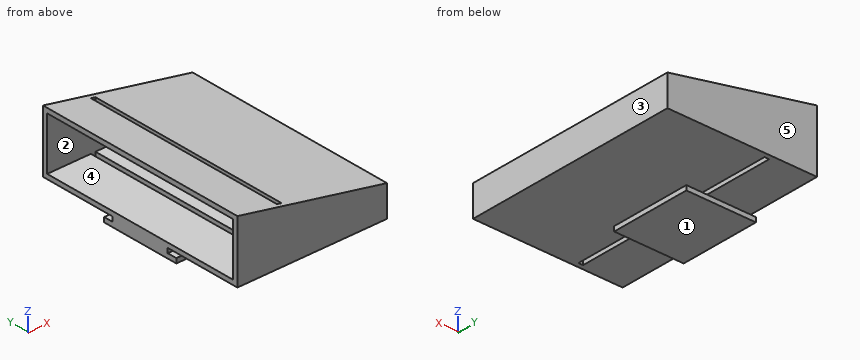
from build123d import *

# Parameters (mm, degrees)
SKETCH1_W           = 2.9
SKETCH1_H           = 19.8
BOSS_EXTRUDE1_DEPTH = 1.5
SKETCH2_W           = 22.5
SKETCH2_H           = 26
BOSS_EXTRUDE3_DEPTH = 1.5
BOSS_EXTRUDE4_DEPTH = 20
CUT_EXTRUDE1_DEPTH  = 70
CUT_EXTRUDE2_START  = -35
CUT_EXTRUDE2_DEPTH  = 33.5
CUT_EXTRUDE3_REACH  = 80.921
SKETCH6_W           = 1.5
SKETCH6_H           = 67


with BuildPart() as part:
    # Sketch1 → Boss-Extrude1 (new body)
    with BuildSketch(Plane.XY):
        with Locations((-45.437495374, 25.25)):
            Rectangle(SKETCH1_W, SKETCH1_H)
    extrude(amount=-BOSS_EXTRUDE1_DEPTH)

    # Sketch2 → Boss-Extrude3 (add)
    with BuildSketch(Plane(origin=(0, 0, -1.5), x_dir=(-1, 0, 0), z_dir=(0, 0, -1))):
        with Locations((35.637495374, 25.25)):
            Rectangle(SKETCH2_W, SKETCH2_H)
    extrude(amount=BOSS_EXTRUDE3_DEPTH)

    # Sketch3 → Boss-Extrude4 (add)
    with BuildSketch(Plane.XY):
        Polygon((-46.887495374, 15.25), (-46.887495374, 35.25), (-46.887495374, 60.25), (1.5, 60.25), (1.5, -9.75), (-46.887495374, -9.75), align=None)
    extrude(amount=BOSS_EXTRUDE4_DEPTH)

    # Sketch4 → Cut-Extrude1 (cut)
    with BuildSketch(Plane.XZ.offset(9.75)):
        Polygon((-46.887495374, 20), (1.5, 10), (1.5, 20), align=None)
    extrude(amount=-CUT_EXTRUDE1_DEPTH, mode=Mode.SUBTRACT)

    # Sketch5 → Cut-Extrude2 (cut)
    with BuildSketch(Plane.XZ.offset(9.75).offset(CUT_EXTRUDE2_START)):
        Polygon((0, 1.5), (0, 8.778299559), (-46.887495374, 18.468302113), (-46.887495374, 1.5), align=None)
    cut_extrude2 = extrude(amount=CUT_EXTRUDE2_DEPTH, mode=Mode.SUBTRACT)

    # Mirror1: Cut-Extrude2 across plane
    add(cut_extrude2.mirror(Plane.ZX.offset(25.25)), mode=Mode.SUBTRACT)

    # Cut-Extrude3: up to this plane
    cut_extrude3_end = Plane(origin=(-46.887495374, 109.660016278, 20), z_dir=(-0.20238811385578315, 0, -0.9793053922908311))
    # Sketch6 → Cut-Extrude3 (cut, up to the surface)
    with BuildSketch(Plane(origin=(0, 0, 0), x_dir=(-1, 0, 0), z_dir=(0, 0, -1)), mode=Mode.PRIVATE) as cut_extrude3_sk1:
        with Locations((32.02, 25.25)):
            Rectangle(SKETCH6_W, SKETCH6_H)
    cut_extrude3_tool1 = split(extrude(cut_extrude3_sk1.sketch, amount=-CUT_EXTRUDE3_REACH, mode=Mode.PRIVATE), bisect_by=cut_extrude3_end, keep=Keep.BOTH, mode=Mode.PRIVATE)
    add(cut_extrude3_tool1.solids().sort_by_distance((-32.02, 25.25, 0))[0], mode=Mode.SUBTRACT)


solid = part.part
Geometry check sheet. Reference: the model listing, model coordinates, mm. Face numbers are marked on the shaded views. A direction names the side the tool comes from. Round coordinates to 2 decimals unless told otherwise and drop trailing zeros. Write each loop counter-clockwise with the first axis right and the second up, starting at its lowest first coordinate (ties: lowest second). Pieces come first, ordered by that corner, then holes. Notation, with made-up numbers: (41, 29) -> (58, 29) arc R13 cw to (58, 33) -> close; hole circle Ø4 at (11, -28.75). An arc over 180 degrees is marked (long way). One line per item, written item: value. Start each with the question number.
(1) Cross-section at A-A, the plane y = 27.5. Record the cut outline in (x, z).
(2) Cross-section at D-D, the plane x = -8. Record the cut outline in (y, z).
(3) Access from +Z, -Z, +X, -X, +Y, -Y to the whole of each face (thin tool, end or side, straight path). Record for the marked faces 4 and 5.
(4) Scan lines: line 1 (Y direction, x = -30.5, z = 8); line 2 (X direction, y = 35.5, z = 1); line 3 (Z direction, x = -37, y = 41.5). Record each from-to range of solid material in increasing order. Write a range as [from, to].
(5) Cross-section at B-B, the plane y = 37. Record the cut outline in (x, z).
(6) Draft check along Z on the marked faces 1, 2 and 3. Enter one of: +Z half, -Z half, draft (parallel to the pull), parting line (faces both ways), or undercut.
(7) Cross-section at C-C, the plane x = -42. Record the cut outline in (y, z), and give its area (3 significant figures).
(8) Go/stop test with flat-tipped pins: pin 1 Ø4 at (x, y) = (-25, 4.5) entering from +Z; pin 2 Ø6 at (x, y) = (-8, 6.5) entering from -Z; pin 3 Ø4 at (y, z) = (38, 4) entering from -X; pin 4 Ø1.2 at (y, z) = (30, -0.5) entering from +X. Record where each tip stops, or that it passes through.
Answer:
1. outline: (-46.89, -3) -> (-24.39, -3) -> (-24.39, -1.5) -> (-43.99, -1.5) -> (-43.99, 0) -> (-32.77, 0) -> (-32.77, 1.5) -> (-46.89, 1.5) -> close; (-46.89, 18.47) -> (-32.77, 15.55) -> (-32.77, 17.08) -> (-46.89, 20) -> close; (-31.27, 0) -> (1.5, 0) -> (1.5, 10) -> (-31.27, 16.77) -> (-31.27, 15.24) -> (0, 8.78) -> (0, 1.5) -> (-31.27, 1.5) -> close
2. outline: (-9.75, 0) -> (60.25, 0) -> (60.25, 11.96) -> (-9.75, 11.96) -> close; hole (-8.25, 1.5) -> (58.75, 1.5) -> (58.75, 10.43) -> (-8.25, 10.43) -> close
3. face 4: -X
3. face 5: +Z, -Z, +X, -X, +Y
4. line 1: [-9.75, -8.25], [58.75, 60.25]
4. line 2: [-46.89, -32.77], [-31.27, 1.5]
4. line 3: [0, 1.5], [16.42, 17.96]
5. outline: (-46.89, -3) -> (-24.39, -3) -> (-24.39, -1.5) -> (-46.89, -1.5) -> close; (-46.89, 0) -> (-32.77, 0) -> (-32.77, 1.5) -> (-46.89, 1.5) -> close; (-46.89, 18.47) -> (-32.77, 15.55) -> (-32.77, 17.08) -> (-46.89, 20) -> close; (-31.27, 0) -> (1.5, 0) -> (1.5, 10) -> (-31.27, 16.77) -> (-31.27, 15.24) -> (0, 8.78) -> (0, 1.5) -> (-31.27, 1.5) -> close
6. face 1: -Z half
6. face 2: undercut
6. face 3: draft
7. outline: (-9.75, 0) -> (60.25, 0) -> (60.25, 18.99) -> (-9.75, 18.99) -> close; (12.25, -3) -> (38.25, -3) -> (38.25, -1.5) -> (12.25, -1.5) -> close; hole (-8.25, 1.5) -> (58.75, 1.5) -> (58.75, 17.46) -> (-8.25, 17.46) -> close
7. area: 299 mm²
8. pin 1: z = 15.89
8. pin 2: z = 0
8. pin 3: x = 0
8. pin 4: x = 1.5
